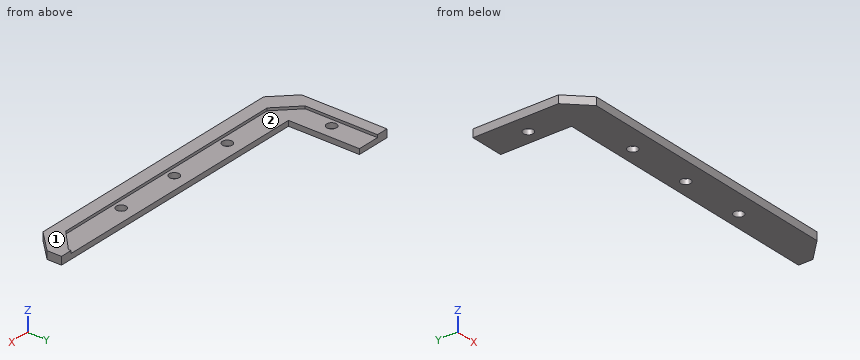
Autodesk Inventor part; units mm, degrees
sketch "Boceto1" plane through (0, 0, 0) normal (0, 0, 1) x (1, 0, 0)
  line L0 (0, 0) -> (107.005, 0)
  line L1 (107.005, 0) -> (107.005, -5.5)
  line L2 (107.005, -5.5) -> (99.0087, -13.4963)
  line L3 (99.0087, -13.4963) -> (-4.9913, -13.4963)
  line L4 (-4.9913, -13.4963) -> (-12.9876, -5.5)
  line L5 (-12.9876, -5.5) -> (-12.9876, 27)
  line L6 (-12.9876, 27) -> (0, 27)
  line L7 (0, 27) -> (0, 0)
  line L8 (107.0124, -0.0005) -> (107.0124, -5.5005)
  line L9 (107.0124, -5.5005) -> (82.0124, -30.5)
  dimension "d0" = 107.005
  dimension "d1" = 5.5
  dimension "d5" = 32.5
  dimension "d8" = 27
  dimension "d34" = 135
extrude "Extrusión1" add sketch "Boceto1" along normal blind 3
sketch "Boceto2" plane through (0, 0, 3) normal (0, 0, 1) x (1, 0, 0)
  circle A0 centre (-5.5, 12) radius 1.89
  line L0 (0, 27) -> (-12.9876, 27)
  point P0 (0, 0)
  dimension "d11" = 3.78
  dimension "d12" = 15
  dimension "d13" = 5.5
extrude "Extrusión2" cut sketch "Boceto2" against normal through all
sketch "Boceto3" plane through (0, 0, 3) normal (0, 0, 1) x (1, 0, 0)
  circle A0 centre (22.0124, -5.5) radius 1.89
  line L0 (-12.9876, 27) -> (-12.9876, -5.5)
  point P0 (0, 0)
  dimension "d16" = 3.78
  dimension "d17" = 5.5
  dimension "d18" = 35
extrude "Extrusión3" cut sketch "Boceto3" against normal through all
pattern_linear "Patrón rectangular1" count 3 spacing 25 along (1, 0, 0) of "Extrusión3"
sketch "Boceto4" plane through (0, 0, 3) normal (0, 0, 1) x (1, 0, 0)
  line L0 (0, 0) -> (0, 27)
  line L1 (107.005, 0) -> (0, 0)
  line L2 (0, 27) -> (-8.5, 27)
  line L3 (0, 27) -> (-12.9876, 27)
  line L4 (-8.5, 27) -> (-8.5, -0.4998)
  line L5 (-0.4998, -8.5) -> (94.505, -8.5)
  line L6 (94.505, -8.5) -> (102.505, -1)
  line L7 (102.505, -1) -> (102.505, 0)
  line L8 (-8.5, -0.4998) -> (-0.4998, -8.5)
  line L9 (107.005, -5.5) -> (107.005, 0)
  dimension "d24" = 8.5
  dimension "d25" = 8.5
  dimension "d26" = 135
  dimension "d27" = 11.314
  dimension "d28" = 1
  dimension "d30" = 12.5
  dimension "d31" = 4.5
extrude "Extrusión4" cut sketch "Boceto4" against normal blind 1
Input: part model. Units: mm. Frame: model coordinates. Face numbers are marked on the shaded views. Coordinates: 2 decimals unless noted, no trailing zeros. Loops run counter-clockwise (first coordinate to the right, second up) from the corner with the lowest first, then second, coordinate; pieces in that order, holes last.
Q1. Contact query for flat-ended pins moving along their axis: pin 1 (3 mm diameter, centred on x = 72.01, y = -5.5, fed in from +Z); pin 2 (0.5 mm diameter, centred on y = 13.5, z = 2.5, fed in from +X); pin 3 (1 mm diameter, centred on x = 60.5, z = 0.5, fed in from +Y); pin 4 (0.8 mm diameter, centred on x = 28, z = 2.5, fed in from +Y). Output: stop coordinate, or through.
Q2. Material intervals for line 1 (X direction, y = -7, z = 0.1) (3 decimals); line 2 (Y direction, x = 72, z = 0.7); line 3 (X direction, y = 15, z = 1.65), sorted ascending.
Q3. Cut plane D-D (y = -2.5). Output: boundary loops of the cut face in (x, z) (3 decimals).
Q4. Cut plane A-A (z = 1.3). Output: boundary loops of the cut face in (x, y) (3 decimals).
Q5. Draft query along X for the marked faces 1 and 2. Return one class per face: +X half, -X half, draft (parallel to the pull), parting line (faces both ways), or undercut.
Q6. Cut plane C-C (x = 89). Output: boundary loops of the cut face in (y, z), then the cut area to 3 significant figures.
Q7. Cut plane B-B (y = 17). Output: boundary loops of the cut face in (x, z).
Working result:
1. pin 1: passes through
1. pin 2: stops at x = -8.5
1. pin 3: stops at y = 0
1. pin 4: stops at y = -8.5
2. line 1: x = -11.488 to 20.863, 23.162 to 45.863, 48.162 to 70.863, 73.162 to 105.505
2. line 2: y = -13.5 to -7.39, -3.61 to 0
2. line 3: x = -12.99 to 0
3. outline: (-12.988, 0) - (107.005, 0) - (107.005, 3) - (100.905, 3) - (100.905, 2) - (-6.5, 2) - (-6.5, 3) - (-12.988, 3) - close
4. outline: (-12.988, -5.5) - (-4.991, -13.496) - (99.009, -13.496) - (107.005, -5.5) - (107.005, 0) - (0, 0) - (0, 27) - (-12.988, 27) - close; hole circle Ø3.78 at (-5.5, 12); hole circle Ø3.78 at (22.012, -5.5); hole circle Ø3.78 at (47.012, -5.5); hole circle Ø3.78 at (72.012, -5.5)
5. face 1: draft
5. face 2: undercut
6. outline: (-13.5, 0) - (0, 0) - (0, 2) - (-8.5, 2) - (-8.5, 3) - (-13.5, 3) - close
6. area: 32.0 mm2
7. outline: (-12.99, 0) - (0, 0) - (0, 2) - (-8.5, 2) - (-8.5, 3) - (-12.99, 3) - close
